Here's the drawing with two shaded views (mm, measured from the low corner). I have some questions. A direction names the side the tool comes from. Give positions to 0.01 mm unless a question says otherwise; leave off trailing zeros. Write each loop counter-clockwise with the first axis right and the second up, starting at its lowest first coordinate (ties: lowest second). Pieces come first, ordered by that corner, then holes.
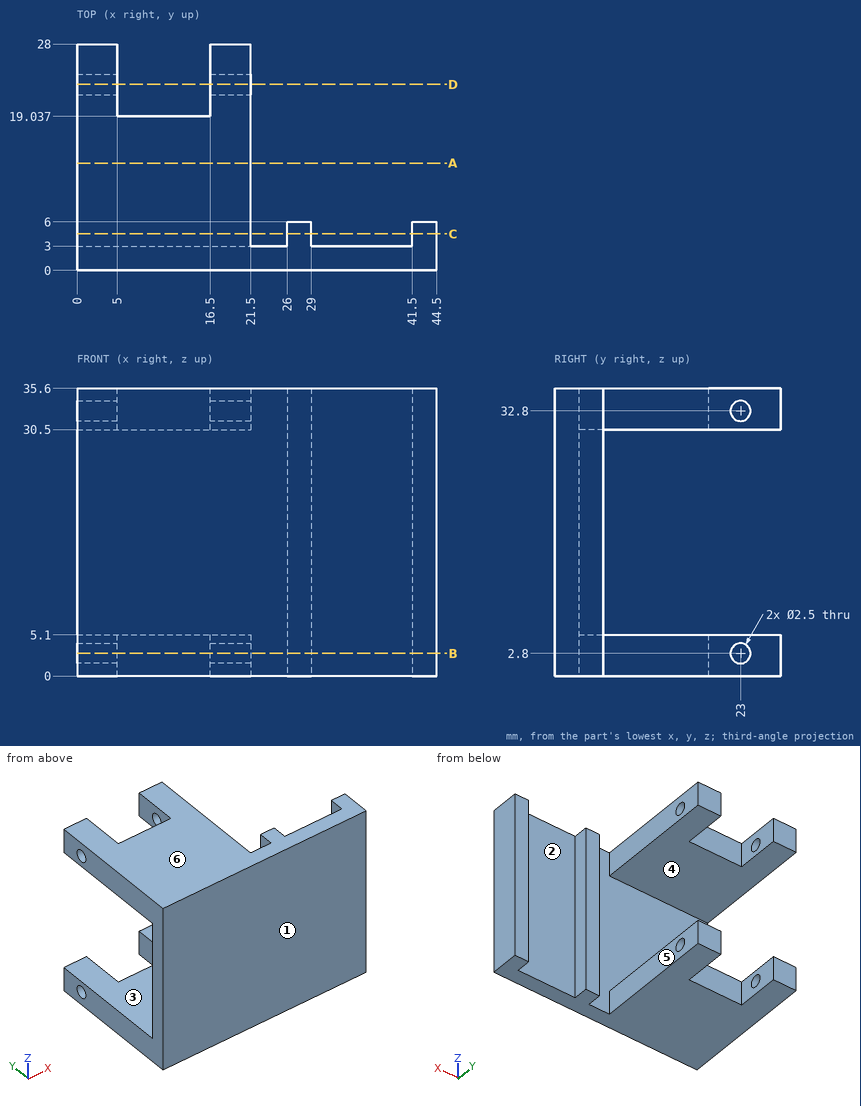
1) If we mould it in two halves opening along Z, with no side actions, what happens to the marked faces 4, 5 and 6? For each: +Z half, -Z half, draft (parallel to the pull), parting line (faces both ways), or undercut.
Values follow:
face 4: undercut
face 5: draft
face 6: +Z half
2) Please list where these lines run through material, in increasing order: L1, parallel to Y at x = 3.5, z = 32.8; L2, parallel to Z at x = 11.5, y = 18.5; L3, parallel to X at y = 11.25, z = 4.
Values follow:
L1: y = 0 to 21.75, 24.25 to 28
L2: z = 0 to 5.1, 30.5 to 35.6
L3: x = 0 to 21.5
3) For the marked faces 1, 2 and 3, which set-ups out of +Z, -Z, +X, -X, +Y, -Y let a thin tool reach every point of the face, with its end or its side?
Values follow:
face 1: +Z, -Z, +X, -X, -Y
face 2: +Z, -Z, +Y
face 3: -X, +Y
4) Suppose I cut it at B-B on z = 2.8. Write out the boundary of the cut face in (x, y), plus the area to 3 significant figures.
Values follow:
outline: (0, 0) - (44.5, 0) - (44.5, 6) - (41.5, 6) - (41.5, 3) - (29, 3) - (29, 6) - (26, 6) - (26, 3) - (21.5, 3) - (21.5, 21.75) - (16.5, 21.75) - (16.5, 19.04) - (5, 19.04) - (5, 21.75) - (0, 21.75) - close; (0, 24.25) - (5, 24.25) - (5, 28) - (0, 28) - close; (16.5, 24.25) - (21.5, 24.25) - (21.5, 28) - (16.5, 28) - close
area: 561 mm2
5) For pin 1 Ø5.5 at (y, z) = (25, 2.5) entering from +X; pin 2 Ø3.5 at (x, z) = (27.5, 10.5) entering from +Y; pin 3 Ø1.5 at (x, z) = (8.5, 33.5) entering from +Y, each with a flat end and sliding along its axis, tell me the tip position at first contact or that it passes through.
Values follow:
pin 1: stops at x = 21.5
pin 2: stops at y = 6
pin 3: stops at y = 19.04
6) Suppose I cut it at D-D on y = 23. State how many separate pieces and enclosed holes the cut face has, plus the area to 3 significant figures.
Values follow:
separate pieces: 8
enclosed holes: 0
area: 52.0 mm2
7) Suppose I cut it at A-A on y = 13.25. Write out the boundary of the cut face in (x, z), plus the area to 3 significant figures.
Values follow:
outline: (0, 0) - (21.5, 0) - (21.5, 5.1) - (0, 5.1) - close; (0, 30.5) - (21.5, 30.5) - (21.5, 35.6) - (0, 35.6) - close
area: 219 mm2
8) Suppose I cut it at C-C on y = 4.5. Write out the boundary of the cut face in (x, z), plus the area to 3 significant figures.
Values follow:
outline: (0, 0) - (21.5, 0) - (21.5, 5.1) - (0, 5.1) - close; (0, 30.5) - (21.5, 30.5) - (21.5, 35.6) - (0, 35.6) - close; (26, 0) - (29, 0) - (29, 35.6) - (26, 35.6) - close; (41.5, 0) - (44.5, 0) - (44.5, 35.6) - (41.5, 35.6) - close
area: 433 mm2
